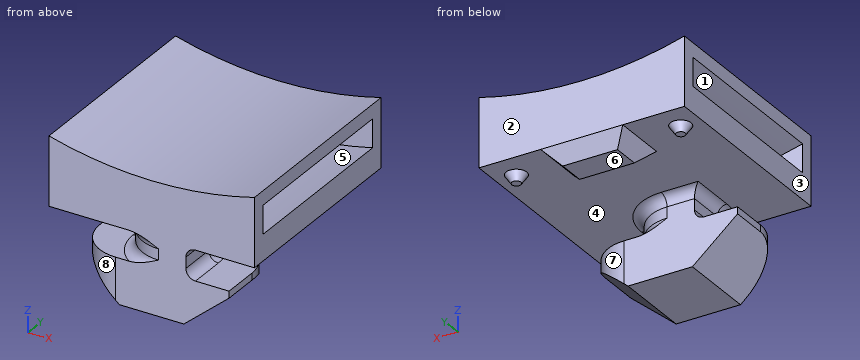
from build123d import *

# Parameters (mm, degrees)
BOSS_EXTRUDE1_DEPTH           = 7.5
CUT_EXTRUDE2_DEPTH            = 9.3
FILLET1_R                     = 3
FILLET2_R                     = 0.7
SKETCH3_W                     = 6
SKETCH3_H                     = 4
BOSS_EXTRUDE2_DEPTH           = 1
BOSS_EXTRUDE2_TAPER           = 45
SKETCH5_R                     = 0.75
BOSS_EXTRUDE3_DEPTH           = 0.6
BOSS_EXTRUDE3_DRAFT           = 35
BOSS_EXTRUDE3_PROFILE_2_DEPTH = 0.6
BOSS_EXTRUDE3_PROFILE_2_DRAFT = 35
CUT_EXTRUDE3_DEPTH            = 6.5


with BuildPart() as part:
    # Sketch1 → Boss-Extrude1 (new, symmetric)
    with BuildSketch(Plane(origin=(0, 0, 0), x_dir=(1, 0, 0), z_dir=(0, 1, 0))):
        with BuildLine():
            Line((-2.35, 5.5), (2.35, 5.5))
            Line((2.35, 5.5), (5.65, 2.7))
            Line((5.65, 2.7), (5.65, 2.2))
            Line((5.65, 2.2), (2.5, 2.2))
            Line((2.5, 2.2), (2.5, 0))
            Line((2.5, 0), (7.5, 0))
            Line((7.5, 0), (7.5, -5))
            ThreePointArc((7.5, -5), (0, -4), (-7.5, -5))
            Line((-7.5, -5), (-7.5, 0))
            Line((-7.5, 0), (-2.5, 0))
            Line((-2.5, 0), (-2.5, 2.2))
            Line((-2.5, 2.2), (-5.65, 2.2))
            Line((-5.65, 2.2), (-5.65, 2.7))
            Line((-5.65, 2.7), (-2.35, 5.5))
        make_face()
    extrude(amount=BOSS_EXTRUDE1_DEPTH, both=True)

    # Sketch2 → Cut-Extrude2 (cut)
    with BuildSketch(Plane(origin=(0, 7.5, 0), x_dir=(1, 0, 0), z_dir=(0, 1, 0))):
        Polygon((-2.5, 0), (2.5, 0), (2.5, 2.2), (5.65, 2.2), (5.65, 2.7), (2.35, 5.5), (-2.35, 5.5), (-5.65, 2.7), (-5.65, 2.2), (-2.5, 2.2), align=None)
    extrude(amount=-CUT_EXTRUDE2_DEPTH, mode=Mode.SUBTRACT)

    # Fillet1
    fillet1_edges = [part.edges().sort_by_distance(p)[0] for p in [
        (-2.5, -7.5, -1.1),
        (-5.65, -7.5, -2.45),
        (5.65, -1.8, -2.45),
        (2.5, -1.8, -1.1),
    ]]
    fillet(fillet1_edges, radius=FILLET1_R)

    # Fillet2
    # the kernel refuses this fillet: 0.7 mm, written as the material it adds along each edge
    with BuildSketch(Plane(origin=(-2.5, -4.5, 0), x_dir=(0, 0, -1), z_dir=(0, 1, 0)), Plane(origin=(-2.5, -1.8, -2.2), x_dir=(0, 0, 1), z_dir=(0, -1, 0)), Plane(origin=(2.5, -4.8, -2.2), x_dir=(1, 0, 0), z_dir=(0, -1, 0)), Plane(origin=(2.5, -4.8, 0), x_dir=(0, 0, -1), z_dir=(0, -1, 0))) as fillet2_piece_1:
        with BuildLine():
            CenterArc((FILLET2_R, FILLET2_R), FILLET2_R, 180, 90)
            Line((0, FILLET2_R), (0, 0))
            Line((0, 0), (FILLET2_R, 0))
        make_face()
    extrude(amount=2.7)
    with BuildSketch(Plane(origin=(-2.5, -1.8, 0), x_dir=(0, 0, -1), z_dir=(1, 0, 0))) as fillet2_piece_2:
        with BuildLine():
            CenterArc((FILLET2_R, FILLET2_R), FILLET2_R, 180, 90)
            Line((0, FILLET2_R), (0, 0))
            Line((0, 0), (FILLET2_R, 0))
        make_face()
    extrude(amount=2)
    with BuildSketch(Plane(origin=(0.5, -4.5, 0), x_dir=(-1, 0, 0), z_dir=(0, 1, 0))) as fillet2_piece_3_section:
        with BuildLine():
            CenterArc((3 + FILLET2_R, -FILLET2_R), FILLET2_R, 90, 90)
            Line((3 + FILLET2_R, 0), (3, 0))
            Line((3, 0), (3, -FILLET2_R))
        make_face()
    fillet2_piece_3 = revolve(axis=Axis((0.5, -4.5, 0), (0, 0, 1)), revolution_arc=146.841139064, mode=Mode.PRIVATE)
    fillet2_piece_3 = split(fillet2_piece_3, bisect_by=Plane(origin=(2.5, -4.5, 0), z_dir=(-1, 0, 0)), keep=Keep.TOP, mode=Mode.PRIVATE)
    fillet2_piece_3 = split(fillet2_piece_3, bisect_by=Plane(origin=(0.5, -7.5, 0), z_dir=(0, 1, 0)), keep=Keep.TOP, mode=Mode.PRIVATE)
    add(fillet2_piece_3)
    with BuildSketch(Plane(origin=(0.5, -4.5, -2.2), x_dir=(-1, 0, 0), z_dir=(0, 1, 0))) as fillet2_piece_4_section:
        with BuildLine():
            CenterArc((3 + FILLET2_R, FILLET2_R), FILLET2_R, 180, 90)
            Line((3, FILLET2_R), (3, 0))
            Line((3, 0), (3 + FILLET2_R, 0))
        make_face()
    fillet2_piece_4 = revolve(axis=Axis((0.5, -4.5, -2.2), (0, 0, 1)), revolution_arc=146.841139064, mode=Mode.PRIVATE)
    fillet2_piece_4 = split(fillet2_piece_4, bisect_by=Plane(origin=(2.5, -4.5, -2.2), z_dir=(-1, 0, 0)), keep=Keep.TOP, mode=Mode.PRIVATE)
    fillet2_piece_4 = split(fillet2_piece_4, bisect_by=Plane(origin=(0.5, -7.5, -2.2), z_dir=(0, 1, 0)), keep=Keep.TOP, mode=Mode.PRIVATE)
    add(fillet2_piece_4)
    with BuildSketch(Plane(origin=(-0.5, -4.8, 0), x_dir=(1, 0, 0), z_dir=(0, -1, 0))) as fillet2_piece_5:
        with BuildLine():
            CenterArc((3 + FILLET2_R, -FILLET2_R), FILLET2_R, 90, 90)
            Line((3 + FILLET2_R, 0), (3, 0))
            Line((3, 0), (3, -FILLET2_R))
        make_face()
    revolve(axis=Axis((-0.5, -4.8, 0), (0, 0, 1)), revolution_arc=90)
    with BuildSketch(Plane(origin=(-0.5, -4.8, -2.2), x_dir=(1, 0, 0), z_dir=(0, -1, 0))) as fillet2_piece_6_section:
        with BuildLine():
            CenterArc((3 + FILLET2_R, FILLET2_R), FILLET2_R, 180, 90)
            Line((3, FILLET2_R), (3, 0))
            Line((3, 0), (3 + FILLET2_R, 0))
        make_face()
    fillet2_piece_6 = revolve(axis=Axis((-0.5, -4.8, -2.2), (0, 0, 1)), revolution_arc=146.841139064, mode=Mode.PRIVATE)
    fillet2_piece_6 = split(fillet2_piece_6, bisect_by=Plane(origin=(-2.5, -4.8, -2.2), z_dir=(1, 0, 0)), keep=Keep.TOP, mode=Mode.PRIVATE)
    fillet2_piece_6 = split(fillet2_piece_6, bisect_by=Plane(origin=(-0.5, -1.8, -2.2), z_dir=(0, -1, 0)), keep=Keep.TOP, mode=Mode.PRIVATE)
    add(fillet2_piece_6)
    with BuildSketch(Plane(origin=(-2.5, -4.5, 0), x_dir=(0, 0, -1), z_dir=(0, 1, 0))) as fillet2_piece_7a_section:
        with BuildLine():
            CenterArc((FILLET2_R, FILLET2_R), FILLET2_R, 180, 90)
            Line((0, FILLET2_R), (0, 0))
            Line((0, 0), (FILLET2_R, 0))
        make_face()
    fillet2_piece_7a = extrude(amount=4.45, mode=Mode.PRIVATE)
    fillet2_piece_7a = split(fillet2_piece_7a, bisect_by=Plane(origin=(-2.5, -1.8, 0), z_dir=(0, 1, 0)), keep=Keep.TOP, mode=Mode.PRIVATE)
    with BuildSketch(Plane(origin=(-4.25, -1.8, 0), x_dir=(0, 0, -1), z_dir=(1, 0, 0))) as fillet2_piece_7b_section:
        with BuildLine():
            CenterArc((FILLET2_R, FILLET2_R), FILLET2_R, 180, 90)
            Line((0, FILLET2_R), (0, 0))
            Line((0, 0), (FILLET2_R, 0))
        make_face()
    fillet2_piece_7b = extrude(amount=3.75, mode=Mode.PRIVATE)
    fillet2_piece_7b = split(fillet2_piece_7b, bisect_by=Plane(origin=(-2.5, -1.8, 0), z_dir=(-1, 0, 0)), keep=Keep.TOP, mode=Mode.PRIVATE)
    fillet2_piece_7 = fillet2_piece_7a & fillet2_piece_7b
    add(fillet2_piece_7)

    # Sketch3 → Boss-Extrude2 (add)
    with BuildSketch(Plane(origin=(0, 0, 0), x_dir=(-1, 0, 0), z_dir=(0, 0, -1))):
        with Locations((0, 5.5)):
            Rectangle(SKETCH3_W, SKETCH3_H)
    extrude(amount=BOSS_EXTRUDE2_DEPTH, taper=BOSS_EXTRUDE2_TAPER)


with BuildPart() as boss_extrude3_tool:
    # Sketch5 → Boss-Extrude3 (with draft: the straight prism first)
    with BuildSketch(Plane(origin=(0, 0, 0), x_dir=(-1, 0, 0), z_dir=(0, 0, -1))):
        with Locations((6, 5.5)):
            Circle(SKETCH5_R)
    extrude(amount=BOSS_EXTRUDE3_DEPTH)
    # Boss-Extrude3: the draft: its side faces are tilted about the plane it starts from
    boss_extrude3_sides = [boss_extrude3_tool.faces().sort_by_distance(p)[0] for p in [
        (-5.25, 5.5, -0.3),
    ]]
    draft(boss_extrude3_sides, Plane(origin=(0, 0, 0), x_dir=(-1, 0, 0), z_dir=(0, 0, -1)), BOSS_EXTRUDE3_DRAFT)


with BuildPart() as part_1:
    add(part.part)

    # Boss-Extrude3: add boss_extrude3_tool
    add(boss_extrude3_tool.part)


with BuildPart() as boss_extrude3_profile_2_tool:
    # Sketch5 → Boss-Extrude3 profile 2 (with draft: the straight prism first)
    with BuildSketch(Plane(origin=(0, 0, 0), x_dir=(-1, 0, 0), z_dir=(0, 0, -1))):
        with Locations((-6, 5.5)):
            Circle(SKETCH5_R)
    extrude(amount=BOSS_EXTRUDE3_PROFILE_2_DEPTH)
    # Boss-Extrude3 profile 2: the draft: its side faces are tilted about the plane it starts from
    boss_extrude3_profile_2_sides = [boss_extrude3_profile_2_tool.faces().sort_by_distance(p)[0] for p in [
        (6.75, 5.5, -0.3),
    ]]
    draft(boss_extrude3_profile_2_sides, Plane(origin=(0, 0, 0), x_dir=(-1, 0, 0), z_dir=(0, 0, -1)), BOSS_EXTRUDE3_PROFILE_2_DRAFT)


with BuildPart() as part_2:
    add(part_1.part)

    # Boss-Extrude3 profile 2: add boss_extrude3_profile_2_tool
    add(boss_extrude3_profile_2_tool.part)

    # Sketch6 → Cut-Extrude3 (cut, symmetric)
    with BuildSketch(Plane(origin=(0, 0, 0), x_dir=(1, 0, 0), z_dir=(0, 1, 0))):
        with BuildLine():
            Line((-7.5, -1.902196987), (-7.5, -3.965086794))
            ThreePointArc((-7.5, -3.965086794), (0, -3), (7.5, -3.965086794))
            Line((7.5, -3.965086794), (7.5, -1.902196987))
            ThreePointArc((7.5, -1.902196987), (0, -1), (-7.5, -1.902196987))
        make_face()
    extrude(amount=CUT_EXTRUDE3_DEPTH, both=True, mode=Mode.SUBTRACT)


solid = part_2.part
Geometry check sheet. Reference: the model listing, model coordinates, mm. Face numbers are marked on the shaded views. A direction names the side the tool comes from. Round coordinates to 2 decimals unless told otherwise and drop trailing zeros. Order: outer loops, then holes, each group sorted by start corner. A loop starts at its lowest first (then second) coordinate and runs counter-clockwise, first axis right, second up. Notation, with made-up numbers: M 79.5,-30.5 L 107.5,-30.5 A27 ccw 107.5,-6.5 Z; hole C -4.5,73 d10. An arc over 180 degrees is marked long. Answer in a Markdown table with one row per item.
(1) Sectioned sample at D-D, the plane x = -6. Record the cut outline in (y, z), and give its area (3 significant figures).
Responses:
| item | result |
|---|---|
| outline | M -7.5,0 L 4.75,0 L 5.17,-0.6 L 5.83,-0.6 L 6.25,0 L 7.5,0 L 7.5,4.64 L -7.5,4.64 Z; hole M -6.5,1.57 L 6.5,1.57 L 6.5,3.61 L -6.5,3.61 Z |
| area | 43.7 mm² |
(2) Sectioned sample at A-A, the plane x = -3.5. Record the cut outline in (y, z).
Responses:
| item | result |
|---|---|
| outline | M -7.5,0 L 7.5,0 L 7.5,4.21 L -7.5,4.21 Z; M -7.38,-4.52 L -1.8,-4.52 L -1.8,-2.2 L -7.38,-2.2 Z; hole M -6.5,1.19 L 6.5,1.19 L 6.5,3.21 L -6.5,3.21 Z |
(3) Sectioned sample at B-B, the plane y = 0.25. Record the cut outline in (x, z) (3 decimals), and give its area (3 significant figures).
Responses:
| item | result |
|---|---|
| outline | M -7.5,0 L 7.5,0 L 7.5,1.902 A31.625 cw -7.5,1.902 Z; M -7.5,3.965 A29.625 ccw 7.5,3.965 L 7.5,5 A28.625 cw -7.5,5 Z |
| area | 34.7 mm² |
(4) Draft check along Y on the marked faces 1, 2, 3 and 4. Enter one of: released by +Y, released by -Y, zero draft, split by the parting line, or undercut.
Responses:
| item | result |
|---|---|
| face 1 | undercut |
| face 2 | released by +Y |
| face 3 | zero draft |
| face 4 | undercut |
(5) Go/stop test with flat-tipped pins: P1, Ø1.5, axis at x = 5, y = -5, coming from the +Z side; P2, Ø0.6, axis at y = -7, z = -1, coming from the +X side; P3, Ø0.7, axis at x = -6, y = 5.5, coming from the -Z side. Record where each tip stops, or that it passes through.
Responses:
| item | result |
|---|---|
| P1 | stops at z = 4.58 |
| P2 | stops at x = 2.5 |
| P3 | stops at z = -0.6 |
(6) Tool access check on the marked faces 5, 6, 7 and 8. Record the directions out of +Z, -Z, +X, -X, +Y, -Y that give a thin tool (end or side, any length) a straight path to the whole face; none if there is none.
Responses:
| item | result |
|---|---|
| face 5 | none |
| face 6 | -Z, +X, -X, +Y |
| face 7 | -Z, +X, +Y |
| face 8 | -Z, -X, -Y |
(7) Sectioned sample at C-C, the plane x = 3.75. Record the cut outline in (y, z).
Responses:
| item | result |
|---|---|
| outline | M -7.5,-4.31 L -2.01,-4.31 L -2.01,-2.2 L -7.5,-2.2 Z; M -7.5,0 L 7.5,0 L 7.5,4.25 L -7.5,4.25 Z; hole M -6.5,1.22 L 6.5,1.22 L 6.5,3.24 L -6.5,3.24 Z |
(8) Scan lines: probe 1 along Y at (x, z) = (4.75, 2.5); probe 2 along Z at (x, y) = (0.5, -3.25); probe 3 along Z at (x, y) = (1.5, -2). Record each from-to range of solid material in increasing order. Write a range as from..to.
Responses:
| item | result |
|---|---|
| probe 1 | y = -7.5..-6.5, 6.5..7.5 |
| probe 2 | z = -5.5..1, 3..4 |
| probe 3 | z = -5.5..-2.15, -0.05..1.04, 3.04..4.04 |
